The drawing under review shows one solid part. Ordinate dimensions are in mm from its lowest x, y, z. A direction names the side the tool comes from. Coordinates: 2 decimals unless noted, no trailing zeros. Order: outer loops, then holes, each group sorted by start corner. A loop starts at its lowest first (then second) coordinate and runs counter-clockwise, first axis right, second up. Notation, with made-up numbers: (32, -16.5) - (73, -16.5) arc R32 cw to (73, 11.5) - close; hole circle Ø8 at (77.5, 8). An arc over 180 degrees is marked (long way). Answer in a Markdown table with one row per item.
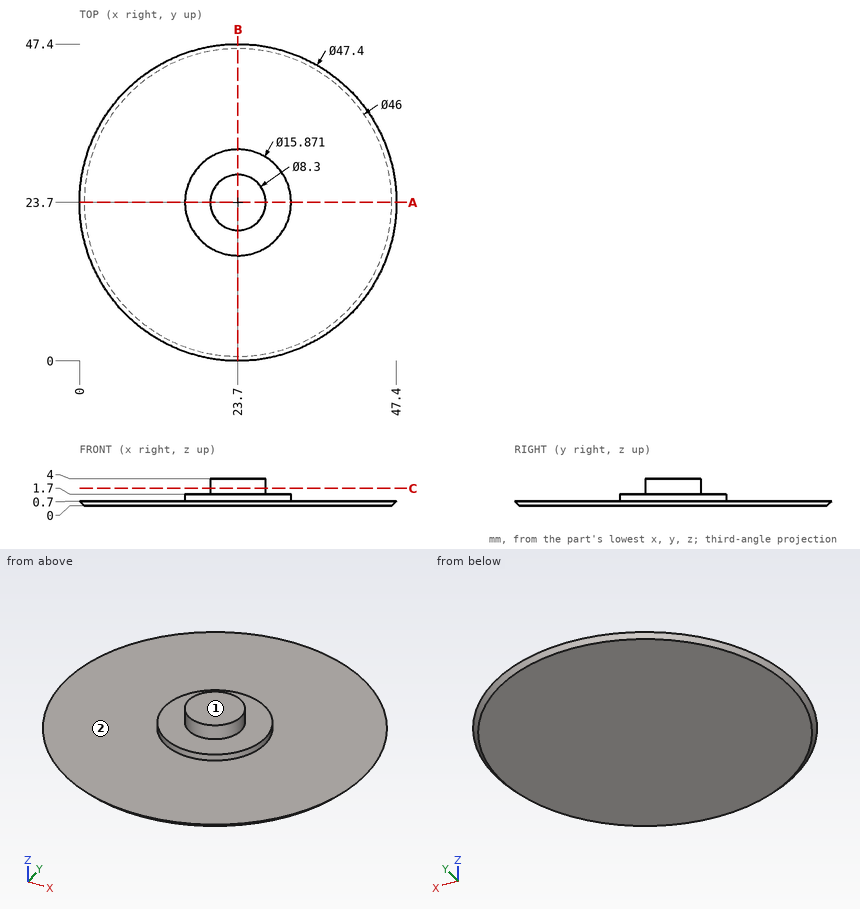
Item 1: Clearance check with flat-ended pins moving along their axes: pin 1 Ø1 at (x, z) = (9.5, 1) entering from -Y; pin 2 Ø14 at (x, y) = (18, 19.5) entering from +Z. State where each tip first meets the part, or that it passes through.
Check values:
| item | result |
|---|---|
| pin 1 | y = 4.43 |
| pin 2 | z = 4 |
Item 2: To check wall thickness, follow line 1 (Z direction, x = 45, y = 22.5); line 2 (Y direction, x = 24.5, z = 3.45); line 3 (Y direction, x = 27, z = 3.1). State the ranges of each line that lie inside material, in increasing order. Write a range as from..to.
Check values:
| item | result |
|---|---|
| line 1 | 0..0.7 |
| line 2 | 19.63..27.77 |
| line 3 | 21.18..26.22 |
Item 3: We need section C-C, the plane z = 2.6. Write out the cut boundary in (x, y), then the cut area to 3 significant figures.
Check values:
| item | result |
|---|---|
| outline | circle Ø8.3 at (23.7, 23.7) |
| area | 54.1 mm^2 |
Item 4: Tool access review of the marked faces 1 and 2: name each direction out of +Z, -Z, +X, -X, +Y, -Y from which nothing blocks a thin tool from reaching the whole face with its end or side.
Check values:
| item | result |
|---|---|
| face 1 | +Z, +X, -X, +Y, -Y |
| face 2 | +Z |
Item 5: We need section A-A, the plane y = 23.7. Write out the cut boundary in (x, z).
Check values:
| item | result |
|---|---|
| outline | (0, 0.7) - (0.7, 0) - (46.7, 0) - (47.4, 0.7) - (31.64, 0.7) - (31.64, 1.7) - (27.85, 1.7) - (27.85, 4) - (19.55, 4) - (19.55, 1.7) - (15.76, 1.7) - (15.76, 0.7) - close |
